Verification items for the finished model (mm, model axes). A direction names the side the tool comes from. Round coordinates to 2 decimals unless told otherwise and drop trailing zeros. Order: outer loops, then holes, each group sorted by start corner. A loop starts at its lowest first (then second) coordinate and runs counter-clockwise, first axis right, second up. Notation, with made-up numbers: (-3.75, 26.25) -> (44.25, 26.25) arc R10 cw to (44.25, 36.25) -> close; hole circle Ø11 at (63, 14). An arc over 180 degrees is marked (long way). Put each result on its own line as item: value.
```python
from build123d import *

# Parameters (mm, degrees)
SKETCH1_W                                        = 36
SKETCH1_H                                        = 50
BOSS_EXTRUDE1_DEPTH                              = 69.85
CBORE_FOR_1_2_SOCKET_HEAD_CAP_SCREW1_D           = 13.89126
CBORE_FOR_1_2_SOCKET_HEAD_CAP_SCREW1_CBORE_D     = 20.6375
CBORE_FOR_1_2_SOCKET_HEAD_CAP_SCREW1_CBORE_DEPTH = 27.94
CUT_EXTRUDE1_DEPTH                               = 4
CUT_EXTRUDE2_DEPTH                               = 3
CUT_EXTRUDE4_DEPTH                               = 4.25
CUT_EXTRUDE5_DEPTH                               = 3
SKETCH10_R                                       = 6
CUT_EXTRUDE6_DEPTH                               = 5
FILLET1_R                                        = 0.1
FILLET2_R                                        = 0.254


with BuildPart() as part:
    # Sketch1 → Boss-Extrude1 (new body, symmetric)
    with BuildSketch(Plane(origin=(0, 0, 0), x_dir=(0, 0, -1), z_dir=(1, 0, 0))):
        Rectangle(SKETCH1_W, SKETCH1_H)
    extrude(amount=BOSS_EXTRUDE1_DEPTH, both=True)

    # CBORE for 1/2 Socket Head Cap Screw1 (through all)
    with Locations(Plane.XY.offset(18)):
        with Locations((-49.2125, -1.124), (49.2125, -1.124)):
            CounterBoreHole(CBORE_FOR_1_2_SOCKET_HEAD_CAP_SCREW1_D / 2, CBORE_FOR_1_2_SOCKET_HEAD_CAP_SCREW1_CBORE_D / 2, CBORE_FOR_1_2_SOCKET_HEAD_CAP_SCREW1_CBORE_DEPTH)

    # Sketch5 → Cut-Extrude1 (cut)
    with BuildSketch(Plane(origin=(0, 25, 0), x_dir=(1, 0, 0), z_dir=(0, 1, 0))):
        with BuildLine():
            Line((-65.85, -18), (-45.85, -18))
            Line((-45.85, -18), (-45.85, -11))
            ThreePointArc((-45.85, -11), (-47.85, -9), (-49.85, -11))
            Line((-49.85, -11), (-49.85, -13))
            Line((-49.85, -13), (-61.85, -13))
            Line((-61.85, -13), (-61.85, -11))
            ThreePointArc((-61.85, -11), (-63.85, -9), (-65.85, -11))
            Line((-65.85, -11), (-65.85, -18))
        make_face()
        with BuildLine():
            Line((45.85, -18), (65.85, -18))
            Line((65.85, -18), (65.85, -11))
            ThreePointArc((65.85, -11), (63.85, -9), (61.85, -11))
            Line((61.85, -11), (61.85, -13))
            Line((61.85, -13), (49.85, -13))
            Line((49.85, -13), (49.85, -11))
            ThreePointArc((49.85, -11), (47.85, -9), (45.85, -11))
            Line((45.85, -11), (45.85, -18))
        make_face()
    extrude(amount=-CUT_EXTRUDE1_DEPTH, mode=Mode.SUBTRACT)

    # Sketch6 → Cut-Extrude2 (cut)
    with BuildSketch(Plane(origin=(0, 25, 0), x_dir=(1, 0, 0), z_dir=(0, 1, 0))):
        with BuildLine():
            Line((-40.85, -18), (-25.358066615, -18))
            ThreePointArc((-25.358066615, -18), (-33.104033308, -12), (-40.85, -18))
        make_face()
        with BuildLine():
            Line((25.358066615, -18), (40.85, -18))
            ThreePointArc((40.85, -18), (33.104033308, -12), (25.358066615, -18))
        make_face()
    extrude(amount=-CUT_EXTRUDE2_DEPTH, mode=Mode.SUBTRACT)

    # Sketch8 → Cut-Extrude4 (cut)
    with BuildSketch(Plane.XY.offset(18)):
        with BuildLine():
            Line((-37.104033308, 22), (-29.104033308, 22))
            Line((-29.104033308, 22), (-29.104033308, 13.5875))
            ThreePointArc((-29.104033308, 13.5875), (-29.569001292, 12.464967985), (-30.691533308, 12))
            Line((-30.691533308, 12), (-35.516533308, 12))
            ThreePointArc((-35.516533308, 12), (-36.639065323, 12.464967985), (-37.104033308, 13.5875))
            Line((-37.104033308, 13.5875), (-37.104033308, 22))
        make_face()
        with BuildLine():
            Line((29.104033308, 22), (37.104033308, 22))
            Line((37.104033308, 22), (37.104033308, 13.5875))
            ThreePointArc((37.104033308, 13.5875), (36.639065323, 12.464967985), (35.516533308, 12))
            Line((35.516533308, 12), (30.691533308, 12))
            ThreePointArc((30.691533308, 12), (29.569001292, 12.464967985), (29.104033308, 13.5875))
            Line((29.104033308, 13.5875), (29.104033308, 22))
        make_face()
    extrude(amount=-CUT_EXTRUDE4_DEPTH, mode=Mode.SUBTRACT)

    # Sketch9 → Cut-Extrude5 (cut)
    with BuildSketch(Plane.XY.offset(18)):
        with BuildLine():
            Line((-16.358066615, 21.25), (-8.358066615, 21.25))
            ThreePointArc((-8.358066615, 21.25), (-6.358066615, 19.25), (-4.358066615, 21.25))
            ThreePointArc((-4.358066615, 21.25), (-4.59491081, 23.18220391), (-5.291419603, 25))
            Line((-5.291419603, 25), (-19.424713628, 25))
            ThreePointArc((-19.424713628, 25), (-20.12122242, 23.18220391), (-20.358066615, 21.25))
            ThreePointArc((-20.358066615, 21.25), (-18.358066615, 19.25), (-16.358066615, 21.25))
        make_face()
        with BuildLine():
            Line((5.291419603, 25), (19.424713628, 25))
            ThreePointArc((19.424713628, 25), (20.12122242, 23.18220391), (20.358066615, 21.25))
            ThreePointArc((20.358066615, 21.25), (18.358066615, 19.25), (16.358066615, 21.25))
            Line((16.358066615, 21.25), (8.358066615, 21.25))
            ThreePointArc((8.358066615, 21.25), (6.358066615, 19.25), (4.358066615, 21.25))
            ThreePointArc((4.358066615, 21.25), (4.59491081, 23.18220391), (5.291419603, 25))
        make_face()
    extrude(amount=-CUT_EXTRUDE5_DEPTH, mode=Mode.SUBTRACT)

    # Sketch10 → Cut-Extrude6 (cut)
    with BuildSketch(Plane(origin=(0, 25, 0), x_dir=(1, 0, 0), z_dir=(0, 1, 0))):
        Circle(SKETCH10_R)
    extrude(amount=-CUT_EXTRUDE6_DEPTH, mode=Mode.SUBTRACT)

    # Fillet1
    fillet1_edges = [part.edges().sort_by_distance(p)[0] for p in [
        (-16.358066615, 21.25, 16.5),
        (-8.358066615, 21.25, 16.5),
        (16.358066615, 21.25, 16.5),
        (8.358066615, 21.25, 16.5),
    ]]
    fillet(fillet1_edges, radius=FILLET1_R)

    # Fillet2
    fillet2_edges = [part.edges().sort_by_distance(p)[0] for p in [
        (-61.85, 23, 13),
        (-49.85, 23, 13),
        (49.85, 23, 13),
        (61.85, 23, 13),
    ]]
    fillet(fillet2_edges, radius=FILLET2_R)


solid = part.part
```
Item 1: Depth check by flat-ended pin: pin 1 Ø16 at (x, y) = (49.21, -1.12) entering from +Z; pin 2 Ø1.3 at (x, z) = (-32.5, 16) entering from +Y. Enter the tip coordinate at first touch or a pass-through.
Geometry check:
pin 1: z = -9.94
pin 2: y = 12
Item 2: Sectioned sample at A-A, the plane z = -3.5. Record the boundary of the cut face in (x, y), then the cut area to 3 significant figures.
Geometry check:
outline: (-69.85, -25) -> (69.85, -25) -> (69.85, 25) -> (4.87, 25) -> (4.87, 20) -> (-4.87, 20) -> (-4.87, 25) -> (-69.85, 25) -> close; hole circle Ø20.64 at (-49.21, -1.12); hole circle Ø20.64 at (49.21, -1.12)
area: 6,270 mm2
Item 3: Material ranges on line 1 along X through (y, z) = (-0.5, 16); line 2 along X through (y, z) = (6.5, -5.5); line 3 along X through (y, z) = (23.8, 0), recorded low to high.
Geometry check:
line 1: -69.85 to -59.51, -38.91 to 38.91, 59.51 to 69.85
line 2: -69.85 to -56.17, -42.26 to 42.26, 56.17 to 69.85
line 3: -69.85 to -6, 6 to 69.85
Item 4: Release check for a two-part mould opening along Y. For faces 4 (the face through (56, 21, 14)), 5 (the face through (63.9, 23, 9)), 6 (the face through (-39.37, 1.98, 4.23)) record: pulls with the +Y half, pulls with the -Y half, needs draft (parallel to the pull), parting line crosses it, or undercut.
Geometry check:
face 4: pulls with the +Y half
face 5: needs draft
face 6: undercut
Item 5: Sectioned sample at C-C, the plane y = 1.5. Record the boundary of the cut face in (x, z).
Geometry check:
outline: (-69.85, -18) -> (-55.64, -18) -> (-55.64, -9.94) -> (-59.19, -9.94) -> (-59.19, 18) -> (-69.85, 18) -> close; (-42.78, -18) -> (42.78, -18) -> (42.78, -9.94) -> (39.23, -9.94) -> (39.23, 18) -> (-39.23, 18) -> (-39.23, -9.94) -> (-42.78, -9.94) -> close; (55.64, -18) -> (69.85, -18) -> (69.85, 18) -> (59.19, 18) -> (59.19, -9.94) -> (55.64, -9.94) -> close
Item 6: Sectioned sample at D-D, the plane x = 0. Record the boundary of the cut face in (y, z).
Geometry check:
outline: (-25, -18) -> (25, -18) -> (25, -6) -> (20, -6) -> (20, 6) -> (25, 6) -> (25, 18) -> (-25, 18) -> close
Item 7: Tool access check on faces 1 (the face through (-4.6, 23.2, 16.5)), 2 (the face through (-29.104, 18, 16)), 3 (the face through (1, 0, -18)). Record the directions out of +Z, -Z, +X, -X, +Y, -Y that give a thin tool (end or side, any length) a straight path to the whole face; none if there is none.
Geometry check:
face 1: +Z
face 2: +Z, +Y
face 3: -Z, +X, -X, +Y, -Y
Item 8: Sectioned sample at B-B, the plane x = 47.85. Record the boundary of the cut face in (y, z), then the cut area to 3 significant figures.
Geometry check:
outline: (-25, -18) -> (-7.93, -18) -> (-7.93, -9.94) -> (-11.35, -9.94) -> (-11.35, 18) -> (-25, 18) -> close; (5.69, -18) -> (25, -18) -> (25, 9) -> (21, 9) -> (21, 18) -> (9.1, 18) -> (9.1, -9.94) -> (5.69, -9.94) -> close
area: 1,080 mm2
